Could you check a few things on this model? Use its own coordinates, in mm. A direction names the side the tool comes from. Coordinates: 2 decimals unless noted, no trailing zeros. Order: outer loops, then holes, each group sorted by start corner. A loop starts at its lowest first (then second) coordinate and runs counter-clockwise, first axis right, second up. Notation, with made-up numbers: (66, 0) -> (88, 0) arc R23 ccw to (88, 33) -> close; hole circle Ø8 at (11, 72.25). An arc over 180 degrees is marked (long way). Return JSON: item names as keys, results as strings. Group by question number.
from build123d import *

# Parameters (mm, degrees)
BOSS_EXTRUDE1_DEPTH = 10
SKETCH3_W           = 128
SKETCH3_H           = 86
SKETCH3_W_2         = 66
SKETCH3_H_2         = 212
CUT_EXTRUDE1_DEPTH  = 345.796316686
CUT_EXTRUDE2_DEPTH  = 345.796316686
SKETCH6_W           = 343.5
SKETCH6_H           = 159.021787697
CUT_EXTRUDE3_DEPTH  = 345.796316686
SKETCH7_W           = 86.89559668
SKETCH7_H           = 224.425885746
CUT_EXTRUDE4_DEPTH  = 345.796316686


with BuildPart() as part:
    # Sketch4 → Boss-Extrude1 (new body)
    with BuildSketch(Plane(origin=(0, 0, 0), x_dir=(1, 0, 0), z_dir=(0, 1, 0))):
        with BuildLine():
            Line((-221, 107.5), (95, 107.5))
            ThreePointArc((95, 107.5), (103.838834765, 103.838834765), (107.5, 95))
            Line((107.5, 95), (107.5, -241))
            ThreePointArc((107.5, -241), (103.838834765, -249.838834765), (95, -253.5))
            Line((95, -253.5), (-221, -253.5))
            ThreePointArc((-221, -253.5), (-229.838834765, -249.838834765), (-233.5, -241))
            Line((-233.5, -241), (-233.5, 95))
            ThreePointArc((-233.5, 95), (-229.838834765, 103.838834765), (-221, 107.5))
        make_face()
    extrude(amount=BOSS_EXTRUDE1_DEPTH)

    # Sketch3 → Cut-Extrude1 (cut, through all)
    with BuildSketch(Plane(origin=(0, 0, 0), x_dir=(1, 0, 0), z_dir=(0, 1, 0))):
        with Locations((0, -180.5)):
            Rectangle(SKETCH3_W, SKETCH3_H)
        with Locations((-170.5, -117.5)):
            Rectangle(SKETCH3_W_2, SKETCH3_H_2)
    extrude(amount=CUT_EXTRUDE1_DEPTH, mode=Mode.SUBTRACT)

    # Sketch1 → Cut-Extrude2 (cut, through all)
    with BuildSketch(Plane(origin=(0, 0, 0), x_dir=(1, 0, 0), z_dir=(0, 1, 0))):
        with BuildLine():
            Line((-62.5, -77.5), (62.5, -77.5))
            ThreePointArc((62.5, -77.5), (73.106601718, -73.106601718), (77.5, -62.5))
            Line((77.5, -62.5), (77.5, 62.5))
            ThreePointArc((77.5, 62.5), (73.106601718, 73.106601718), (62.5, 77.5))
            Line((62.5, 77.5), (-62.5, 77.5))
            ThreePointArc((-62.5, 77.5), (-73.106601718, 73.106601718), (-77.5, 62.5))
            Line((-77.5, 62.5), (-77.5, -62.5))
            ThreePointArc((-77.5, -62.5), (-73.106601718, -73.106601718), (-62.5, -77.5))
        make_face()
    extrude(amount=CUT_EXTRUDE2_DEPTH, mode=Mode.SUBTRACT)

    # Sketch6 → Cut-Extrude3 (cut, through all)
    with BuildSketch(Plane(origin=(0, 0, 0), x_dir=(1, 0, 0), z_dir=(0, 1, 0))):
        with Locations((-61.75, 36.875290319)):
            Rectangle(SKETCH6_W, SKETCH6_H)
    extrude(amount=CUT_EXTRUDE3_DEPTH, mode=Mode.SUBTRACT)

    # Sketch7 → Cut-Extrude4 (cut, through all)
    with BuildSketch(Plane(origin=(0, 0, 0), x_dir=(1, 0, 0), z_dir=(0, 1, 0))):
        with Locations((-197.154605401, -141.287057127)):
            Rectangle(SKETCH7_W, SKETCH7_H)
    extrude(amount=CUT_EXTRUDE4_DEPTH, mode=Mode.SUBTRACT)


solid = part.part
Q1. I want a section at B-B on z = 198.5. Please give me the cut outline in (x, y), and give its area (3 significant figures).
Q2. I'm going to push a flat-ended pin straight in: pin 1 Ø3 at (y, z) = (4.5, 193.5) entering from -X. Where does the tip first touch, or does it pass through?
Q3. On a 3-axis mill with a long thin cutter (end or side, diameter ignored), from which of +Z, -Z, +X, -X, +Y, -Y can I reach the whole of each face in a straight line? I mean faces 5 (the flat face through (-137.5, 5, 134)), 6 (the flat face through (-64, 5, 181)), 7 (the cylindrical face through (-73.22, 4.93, 72.99)). Say none if no direction works.
Q4. I want a section at A-A on x = -47. Please give me the cut outline in (y, z).
Q5. I want a section at D-D on z = 133. Please give me the cut outline in (x, y), and give its area (3 significant figures).
Q6. I want a section at C-C on y = 3. Please give me the cut outline in (x, z).
Q7. We'd pull the mould along X, two halves only. Please class faces 1 (the flat face through (-108, 5, 42.636)), 2 (the cylindrical face through (103.935, 4.93, 249.741)), 3 (the flat face through (-1, 5, 223.5)), 4 (the flat face through (-153.707, 5, 239)): pulls with the +X half, pulls with the -X half, needs draft (parallel to the pull), parting line crosses it, or undercut.
Q8. I need wall thicknesses on line 1 along X through (y, z) = (2, 187); line 2 along Z through (x, y) = (-17, 7.25); line 3 along X through (y, z) = (4.5, 132). Which ranges of each line are inside material? Lowest first, please. Write a range as from..to.
Response values:
{
 "1": {"outline": "(-137.5, 0) -> (-64, 0) -> (-64, 10) -> (-137.5, 10) -> close; (64, 0) -> (107.5, 0) -> (107.5, 10) -> (64, 10) -> close", "area": "1,170 mm²"},
 "2": {"pin 1": "stops at x = -137.5"},
 "3": {"face 5": "-Z, -X, +Y, -Y", "face 6": "+Y, -Y", "face 7": "-Z, +Y, -Y"},
 "4": {"outline": "(0, 77.5) -> (10, 77.5) -> (10, 137.5) -> (0, 137.5) -> close; (0, 223.5) -> (10, 223.5) -> (10, 253.5) -> (0, 253.5) -> close"},
 "5": {"outline": "(-137.5, 0) -> (107.5, 0) -> (107.5, 10) -> (-137.5, 10) -> close", "area": "2,450 mm²"},
 "6": {"outline": "(-153.71, 223.5) -> (-137.5, 223.5) -> (-137.5, 42.64) -> (-77.5, 42.64) -> (-77.5, 62.5) arc R15 cw to (-62.5, 77.5) -> (62.5, 77.5) arc R15 cw to (77.5, 62.5) -> (77.5, 42.64) -> (107.5, 42.64) -> (107.5, 241) arc R12.5 ccw to (95, 253.5) -> (-153.71, 253.5) -> close; hole (-64, 137.5) -> (64, 137.5) -> (64, 223.5) -> (-64, 223.5) -> close"},
 "7": {"face 1": "needs draft", "face 2": "pulls with the +X half", "face 3": "undercut", "face 4": "pulls with the -X half"},
 "8": {"line 1": "x = -137.5..-64, 64..107.5", "line 2": "z = 77.5..137.5, 223.5..253.5", "line 3": "x = -137.5..107.5"}
}
